Can you work these out from the model? Positions are in its coordinate system, mm. A direction names the side the tool comes from. Coordinates: 2 decimals unless noted, no trailing zeros. Order: outer loops, then holes, each group sorted by start corner. A loop starts at its lowest first (then second) coordinate and runs counter-clockwise, first axis right, second up. Notation, with made-up numbers: M 62,-26 L 103,-26 A32 ccw 103,7 Z; hole C 1.5,-38.5 d4. An arc over 180 degrees is marked long. Answer as a JSON object with one key per item and string values.
from build123d import *

# Parameters (mm, degrees)
F0_R     = 2.65
F1_DEPTH = 0.95
F3_DEPTH = 3.25
F4_R     = 2.09999
F5_R     = 1.15
F6_DEPTH = 25


# Not quite as in the source:
# - a fillet or chamfer is up to 0.001 mm smaller than in the source, because OpenCascade refuses the exact size


with BuildPart() as f1:
    # F0 (on Top) → F1 (new body)
    with BuildSketch(Plane.XY):
        with BuildLine():
            Line((12.5502312096, 2.65), (17, 2.65))
            Line((17, 2.65), (17, 6.85))
            Line((17, 6.85), (12.5502312096, 6.85))
            ThreePointArc((12.5502312096, 6.85), (11.5247662629, 6.9620131907), (10.5476657796, 7.2927698345))
            Line((10.5476657796, 7.2927698345), (6.75256543, 9.0572301655))
            ThreePointArc((6.75256543, 9.0572301655), (5.7754649467, 9.3879868093), (4.75, 9.5))
            ThreePointArc((4.75, 9.5), (1.3912427894, 8.1087572106), (0, 4.75))
            ThreePointArc((0, 4.75), (1.3912427894, 1.3912427894), (4.75, 0))
            ThreePointArc((4.75, 0), (5.7754649467, 0.1120131907), (6.75256543, 0.4427698345))
            Line((6.75256543, 0.4427698345), (10.5476657796, 2.2072301655))
            ThreePointArc((10.5476657796, 2.2072301655), (11.5247662629, 2.5379868093), (12.5502312096, 2.65))
        make_face()
        with Locations((4.75, 4.75)):
            Circle(F0_R, mode=Mode.SUBTRACT)
    extrude(amount=F1_DEPTH)

    # F2 (on face) → F3 (join)
    with BuildSketch(Plane.XY.offset(0.95)):
        Polygon((17, 2.65), (17, 6.85), (12.5502312096, 6.85), (12.5, 6.85), (12.5, 2.65), (12.5502312096, 2.65), align=None)
    extrude(amount=F3_DEPTH)

    # F4 (radius 2.1 in the source; OpenCascade refuses exactly that, so slightly less here)
    f4_edges = [f1.edges().sort_by_distance(p)[0] for p in [
        (14.75, 6.85, 4.2),
        (14.75, 2.65, 4.2),
    ]]
    fillet(f4_edges, radius=F4_R)

    # F5 (on face) → F6 (cut)
    with BuildSketch(Plane.YZ.offset(17)):
        with Locations((4.75, 2.1)):
            Circle(F5_R)
    extrude(amount=-F6_DEPTH, mode=Mode.SUBTRACT)


solid = f1.part
Item 1: If we mould it in two halves opening along X, with no side actions, what happens to faces 4 (the flat face through (8, 5, 0.95)), 5 (the flat face through (8.68, 8.16, 0.47)), 6 (the cylindrical face through (7.2, 3.74, 0.47))? For each: pulls with the +X half, pulls with the -X half, needs draft (parallel to the pull), parting line crosses it, or undercut.
Answers follow:
{"face 4": "needs draft", "face 5": "pulls with the +X half", "face 6": "undercut"}
Item 2: Which directions (+Z, -Z, +X, -X, +Y, -Y) give clear straight access to the entire face, cutting with the end or side of a thin tool? Please do faces 1 (the flat face through (15, 2.65, 1)), 2 (the flat face through (15, 6.85, 1)), 3 (the flat face through (12.5, 6, 3)).
Answers follow:
{"face 1": "+Z, -Z, +X, -Y", "face 2": "+Z, -Z, +X, +Y", "face 3": "+Z, -X, +Y, -Y"}
Item 3: I want a section at D-D, the plane y = 5.5. Write out the boundary of the cut face in (x, z).
Answers follow:
{"outline": "M 0.06,0 L 2.21,0 L 2.21,0.95 L 0.06,0.95 Z; M 7.29,0 L 17,0 L 17,1.23 L 12.5,1.23 L 12.5,0.95 L 7.29,0.95 Z; M 12.5,2.97 L 17,2.97 L 17,4.06 L 12.5,4.06 Z"}
Item 4: I want a section at C-C, the plane x = 6. Write out the boundary of the cut face in (y, z), plus the area to 3 significant figures.
Answers follow:
{"outline": "M 0.17,0 L 2.41,0 L 2.41,0.95 L 0.17,0.95 Z; M 7.09,0 L 9.33,0 L 9.33,0.95 L 7.09,0.95 Z", "area": "4.27 mm^2"}
Item 5: Please list where these lines run through material, in increasing order: line 1 (Y direction, x = 14.8, z = 2.1); line 2 (Y direction, x = 4.75, z = 0.5); line 3 (X direction, y = 4.75, z = 0.4).
Answers follow:
{"line 1": "y = 2.65 to 3.6, 5.9 to 6.85", "line 2": "y = 0 to 2.1, 7.4 to 9.5", "line 3": "x = 0 to 2.1, 7.4 to 17"}
Item 6: I want a section at B-B, the plane z = 0.7. Write out the boundary of the cut face in (x, y).
Answers follow:
{"outline": "M 6.75,0.44 L 10.55,2.21 A4.75 cw 12.55,2.65 L 17,2.65 L 17,6.85 L 12.55,6.85 A4.75 cw 10.55,7.29 L 6.75,9.06 A4.75 ccw long Z; hole C 4.75,4.75 d5.3"}
Item 7: I'm going to push flat-ended pins straight in: pin 1 (0.6 mm diameter, centred on x = 15, z = 1, fed in from +Y); pin 2 (1 mm diameter, centred on y = 3, z = 2.5, fed in from -X); pin 3 (1.7 mm diameter, centred on x = 15, z = 0.5, fed in from -Y); pin 4 (4 mm diameter, centred on x = 5.5, y = 5.5, fed in from -Z). Where does each tip first touch, or does it pass through?
Answers follow:
{"pin 1": "stops at y = 6.85", "pin 2": "stops at x = 12.5", "pin 3": "stops at y = 2.65", "pin 4": "stops at z = 0"}
